Verification items for the finished model (mm, model axes). A direction names the side the tool comes from. Give positions to 0.01 mm unless a question says otherwise; leave off trailing zeros. Loops run counter-clockwise (first coordinate to the right, second up) from the corner with the lowest first, then second, coordinate; pieces in that order, holes last. Notation, with made-up numbers: M 25,87 L 58,87 A32 cw 58,126 Z; hole C -27.75,-15.5 d8. An arc over 180 degrees is marked long. Use CSV: the item, a comma, the result in double quotes.
from build123d import *

# Parameters (mm, degrees)
SKETCH1_R           = 20
BOSS_EXTRUDE1_DEPTH = 5
SKETCH2_R           = 15
CUT_EXTRUDE1_DEPTH  = 5
CUT_EXTRUDE3_START  = -5
CUT_EXTRUDE3_DEPTH  = 5
SKETCH7_W           = 5
SKETCH7_H           = 80
BOSS_EXTRUDE2_DEPTH = 5
BOSS_EXTRUDE3_DEPTH = 5
SKETCH10_R          = 1.5
CUT_EXTRUDE4_DEPTH  = 5
SKETCH11_R          = 1.5
BOSS_EXTRUDE4_DEPTH = 5


with BuildPart() as part:
    # Sketch1 → Boss-Extrude1 (new body)
    with BuildSketch(Plane(origin=(0, 0, 0), x_dir=(1, 0, 0), z_dir=(0, 1, 0))):
        with Locations(Location((0, 0, 0), (0, 0, 270))):
            Circle(SKETCH1_R)
    extrude(amount=BOSS_EXTRUDE1_DEPTH)

    # Sketch2 → Cut-Extrude1 (cut)
    with BuildSketch(Plane(origin=(0, 5, 0), x_dir=(1, 0, 0), z_dir=(0, 1, 0))):
        with Locations(Location((0, 0, 0), (0, 0, 270))):
            Circle(SKETCH2_R)
    extrude(amount=-CUT_EXTRUDE1_DEPTH, mode=Mode.SUBTRACT)

    # Sketch3 → Cut-Extrude3 (cut)
    with BuildSketch(Plane(origin=(0, 5, 0), x_dir=(1, 0, 0), z_dir=(0, 1, 0)).offset(CUT_EXTRUDE3_START)):
        with BuildLine():
            Line((6.840402867, 18.793852416), (0, 0))
            Line((0, 0), (-20, 0))
            ThreePointArc((-20, 0), (11.471528727, -16.383040886), (6.840402867, 18.793852416))
        make_face()
    extrude(amount=CUT_EXTRUDE3_DEPTH, mode=Mode.SUBTRACT)

    # Sketch7 → Boss-Extrude2 (add)
    with BuildSketch(Plane(origin=(0, 5, 0), x_dir=(1, 0, 0), z_dir=(0, 1, 0))):
        with Locations((-17.5, -40)):
            Rectangle(SKETCH7_W, SKETCH7_H)
    extrude(amount=-BOSS_EXTRUDE2_DEPTH)

    # Sketch9 → Boss-Extrude3 (add)
    with BuildSketch(Plane(origin=(0, 5, 0), x_dir=(1, 0, 0), z_dir=(0, 1, 0))):
        with BuildLine():
            Line((6.840402867, 18.793852416), (5.13030215, 14.095389312))
            ThreePointArc((5.13030215, 14.095389312), (8.33458406, 15.589570505), (6.840402867, 18.793852416))
        make_face()
    extrude(amount=-BOSS_EXTRUDE3_DEPTH)

    # Sketch10 → Cut-Extrude4 (cut)
    with BuildSketch(Plane(origin=(0, 5, 0), x_dir=(1, 0, 0), z_dir=(0, 1, 0))):
        with Locations(Location((5.985352508, 16.444620864, 0), (0, 0, 270))):
            Circle(SKETCH10_R)
    extrude(amount=-CUT_EXTRUDE4_DEPTH, mode=Mode.SUBTRACT)

    # Sketch11 → Boss-Extrude4 (add)
    with BuildSketch(Plane(origin=(0, 5, 0), x_dir=(1, 0, 0), z_dir=(0, 1, 0))):
        with Locations(Location((-17.5, 0, 0), (0, 0, 270))):
            Circle(SKETCH11_R)
    extrude(amount=BOSS_EXTRUDE4_DEPTH)


solid = part.part
(1) Mould release check, pull along X, two halves, no side actions. Record for faces 1 (the cylindrical face through (-16.235, 7.465, 0.806)), 2 (the cylindrical face through (-8.44, 2.54, -12.4)), 3 (the flat face through (-16, 0, 22)): released by +X, released by -X, zero draft, split by the parting line, or undercut.
Calculated:
face 1,"split by the parting line"
face 2,"undercut"
face 3,"zero draft"
(2) Section check A-A on x = -17.5. Record the cut outline in (y, z), plus the area to 3 significant figures.
Calculated:
outline,"M 0,-9.68 L 5,-9.68 L 5,-1.5 L 10,-1.5 L 10,1.5 L 5,1.5 L 5,80 L 0,80 Z"
area,"463 mm²"
(3) Depth check by flat-ended pin: pin 1 Ø3 at (x, y) = (-10.5, 1.5) entering from +Z; pin 2 Ø10 at (x, z) = (-9.5, -9.5) entering from +Y; pin 3 Ø2.5 at (y, z) = (3.5, 47.5) entering from +X. Enter the tip coordinate at first touch or a pass-through.
Calculated:
pin 1,"stops at z = -9"
pin 2,"stops at y = 5"
pin 3,"stops at x = -15"
(4) Scan lines: L1, parallel to Y at x = -15.75, z = 69.5; L2, parallel to X at y = 4.5, z = 31; L3, parallel to X at y = 8.25, z = -1. Record each from-to range of solid material in increasing order. Write a range as from..to.
Calculated:
L1,"y = 0..5"
L2,"x = -20..-15"
L3,"x = -18.62..-16.38"
(5) Section check D-D on x = -13.5. Record the cut outline in (y, z), plus the area to 3 significant figures.
Calculated:
outline,"M 0,-14.76 L 5,-14.76 L 5,-6.54 L 0,-6.54 Z"
area,"41.1 mm²"
(6) Section check B-B on z = 10.5. Record the cut outline in (x, y).
Calculated:
outline,"M -20,0 L -15,0 L -15,5 L -20,5 Z"
(7) Tool access check on faces 4 (the flat face through (-20, 3, 41)), 5 (the flat face through (-15, 3, 41)). Record the directions out of +Z, -Z, +X, -X, +Y, -Y that give a thin tool (end or side, any length) a straight path to the whole face; none if there is none.
Calculated:
face 4,"+Z, -Z, -X, +Y, -Y"
face 5,"+Z, +X, +Y, -Y"
(8) Section check C-C on y = 9. Record the cut outline in (x, z).
Calculated:
outline,"C -17.5,0 d3"
